Check sheet for the modelled part. Datum: model origin and axes. Units: mm. Face numbers are marked on the shaded views. A direction names the side the tool comes from. Give positions to 0.01 mm unless a question says otherwise; leave off trailing zeros. Order: outer loops, then holes, each group sorted by start corner. A loop starts at its lowest first (then second) coordinate and runs counter-clockwise, first axis right, second up.
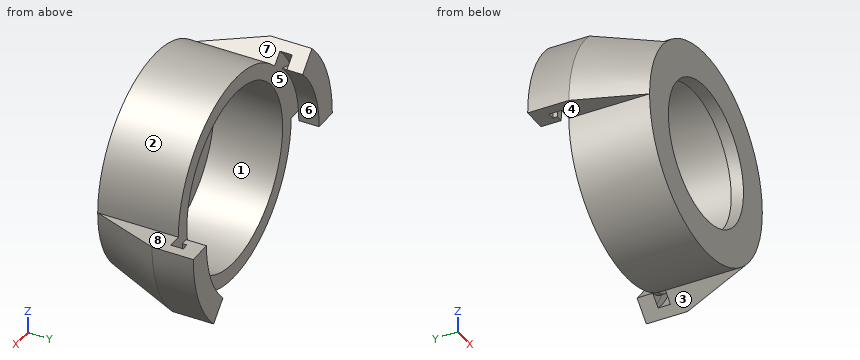
```python
from build123d import *

# Parameters (mm, degrees)
SKETCH_1_R          = 30
SKETCH_1_R_2        = 25.5
EXTRUDE_1_DEPTH     = 23
SKETCH_2_R          = 25.5
SKETCH_2_R_2        = 20
EXTRUDE_2_DEPTH     = 3.5
REVOLVE_1_ANGLE     = 45
CUT_EXTRUDE_1_DEPTH = 1.32
CUT_EXTRUDE_3_DEPTH = 1.32


with BuildPart() as part:
    # 草图1 → 凸台-拉伸1 (new body)
    with BuildSketch(Plane(origin=(0, 0, 0), x_dir=(1, 0, 0), z_dir=(0, 1, 0))):
        with Locations(Location((0, 0, 0), (0, 0, 270))):
            Circle(SKETCH_1_R)
        with Locations(Location((0, 0, 0), (0, 0, 270))):
            Circle(SKETCH_1_R_2, mode=Mode.SUBTRACT)
    extrude(amount=EXTRUDE_1_DEPTH)

    # 草图2 → 凸台-拉伸2 (add)
    with BuildSketch(Plane(origin=(0, 0, 0), x_dir=(1, 0, 0), z_dir=(0, 1, 0))):
        with Locations(Location((0, 0, 0), (0, 0, 270))):
            Circle(SKETCH_2_R)
        with Locations(Location((0, 0, 0), (0, 0, 270))):
            Circle(SKETCH_2_R_2, mode=Mode.SUBTRACT)
    extrude(amount=EXTRUDE_2_DEPTH)

    # 草图3 → 旋转1 (revolve)
    with BuildSketch(Plane.XY):
        Polygon((-30, 0), (-37, 19.23), (-37, 31), (-30, 31), (-30, 25.2), (-32, 25.2), (-32, 26.519651463), (-34, 26.519651463), (-34, 23), (-30, 23), align=None)
    revolve_1 = revolve(axis=Axis((0, 0, 0), (0, 1, 0)), revolution_arc=REVOLVE_1_ANGLE)

    # 镜向1: 旋转1 across plane
    add(revolve_1.mirror(Plane(origin=(0, 0, 0), x_dir=(0.3826834323650901, 0, 0.9238795325112866), z_dir=(0.9238795325112867, 0, -0.38268343236509006))))

    # 草图5 → 切除-拉伸1 (cut)
    with BuildSketch(Plane.XZ.offset(-25.2)):
        with BuildLine():
            Line((-26.405413435, 18.076342033), (-25.672211093, 21.213203436))
            Line((-25.672211093, 21.213203436), (-22.063062958, 24.949941075))
            Line((-22.063062958, 24.949941075), (-17.99117048, 21.673033438))
            Line((-17.99117048, 21.673033438), (-21.213203436, 21.213203436))
            ThreePointArc((-21.213203436, 21.213203436), (-24.149079473, 20.207170096), (-26.405413435, 18.076342033))
        make_face()
    extrude(amount=-CUT_EXTRUDE_1_DEPTH, mode=Mode.SUBTRACT)

    # 草图8 → 切除-拉伸3 (cut)
    with BuildSketch(Plane.XZ.offset(-25.2)):
        with BuildLine():
            Line((26.407763212, -18.072909066), (22.874853187, -24.345219229))
            Line((22.874853187, -24.345219229), (19.318976471, -22.342353909))
            Line((19.318976471, -22.342353909), (21.213203436, -21.213203436))
            ThreePointArc((21.213203436, -21.213203436), (24.150606635, -20.205675758), (26.407763212, -18.072909066))
        make_face()
    extrude(amount=-CUT_EXTRUDE_3_DEPTH, mode=Mode.SUBTRACT)


solid = part.part
```
Q1. Sectioned sample at D-D, the plane x = -12. Record the cut outline in (y, z), plus the area to 3 significant figures.
Q2. Sectioned sample at A-A, the plane y = 27.5. Record the cut outline in (x, z), plus the area to 3 significant figures.
Q3. Tool access check on the marked faces 1, 2, 3, 4 and 5. Record the directions out of +Z, -Z, +X, -X, +Y, -Y that give a thin tool (end or side, any length) a straight path to the whole face; none if there is none.
Q4. Sectioned sample at B-B, the plane x = 0. Record the cut outline in (y, z).
Q5. Go/stop test with flat-tipped pins: P1, Ø2, axis at x = 32, y = 22.5, coming from the +Z side; P2, Ø18, axis at x = -16.5, z = -9.5, coming from the +Y side; P3, Ø2, axis at y = 25.5, z = 9.5, coming from the +X side. Record where each tip stops, or that it passes through.
Q6. Sectioned sample at C-C, the plane y = 22. Record the cut outline in (x, z).
Q7. Draft check along X on the marked faces 6, 7 and 8. Enter one of: pulls with the +X half, pulls with the -X half, needs draft (parallel to the pull), parting line crosses it, or undercut.
Q8. Material ranges on line 1 (Y direction, x = 19, z = -18.5); line 2 (Y direction, x = -22, z = -3.5); line 3 (Z direction, x = -14.5, y = 8), recorded low to high.
Filled in:
1. outline: (0, -27.5) - (23, -27.5) - (23, -22.5) - (3.5, -22.5) - (3.5, -16) - (0, -16) - close; (0, 16) - (3.5, 16) - (3.5, 22.5) - (23, 22.5) - (23, 27.5) - (0, 27.5) - close
1. area: 275 mm2
2. outline: (-37, 0) - (-30, 0) arc R30 cw to (-21.21, 21.21) - (-26.16, 26.16) arc R37 ccw to start; (21.21, -21.21) - (26.16, -26.16) arc R37 ccw to (37, 0) - (30, 0) arc R30 cw to start
2. area: 368 mm2
3. face 1: +Y
3. face 2: +Z, +Y, -Y
3. face 3: -Z, +Y, -Y
3. face 4: -Z, -X, +Y, -Y
3. face 5: none
4. outline: (0, -30) - (23, -30) - (23, -25.5) - (3.5, -25.5) - (3.5, -20) - (0, -20) - close; (0, 20) - (3.5, 20) - (3.5, 25.5) - (23, 25.5) - (23, 30) - (0, 30) - close
5. P1: stops at z = 0
5. P2: stops at y = 23
5. P3: stops at x = -28.1
6. outline: (-37, 0) - (-30, 0) arc R30 ccw to (21.21, -21.21) - (26.16, -26.16) arc R37 ccw to (37, 0) - (30, 0) arc R30 ccw to (-21.21, 21.21) - (-26.16, 26.16) arc R37 ccw to start; hole circle Ø51 at (0, 0)
7. face 6: pulls with the +X half
7. face 7: undercut
7. face 8: needs draft
8. line 1: y = 0 to 23
8. line 2: y = 0 to 3.5
8. line 3: z = -26.26 to -20.98, 20.98 to 26.26
